Input: dimensioned drawing with shaded views. Units: mm. Origin: part minimum x, y, z. A direction names the side the tool comes from. Give positions to 0.01 mm unless a question says otherwise; leave off trailing zeros. Write each loop counter-clockwise with the first axis right and the second up, starting at its lowest first coordinate (ties: lowest second). Pieces come first, ordered by that corner, then holes.
Q1. Section D-D (x = 37.5). Return the cut outline in (y, z).
Q2. Pin query (flat end, axial travel): pin 1 Ø5 at (y, z) = (12, 67) entering from -X; pin 2 Ø1.5 at (x, y) = (29.5, 11) entering from -Z; pin 3 Ø3 at (x, y) = (45.5, 15.5) entering from +Z; pin 4 Ø10 at (x, y) = (33.5, 15.5) entering from +Z. Return the tip coordinate at first contact, or that it passes through.
Q3. Section A-A (x = 30). Return the cut outline in (y, z), plus the area to 3 significant figures.
Q4. Reachability of the marked faces 1, 2 and 3 from +Z, -Z, +X, -X, +Y, -Y: full face, straight path, thin tool, end or side. Return the list, or none.
Q5. Section C-C (z = 60). Return the cut outline in (x, y).
Q6. Line query: line 1 (Z direction, x = 15, y = 0.35); line 2 (Y direction, x = 49, z = 55); line 3 (Z direction, x = 49, y = 8.5). Output: solid intervals per line, ascending.
Q7. Section B-B (y = 9.25). Return the cut outline in (x, z).
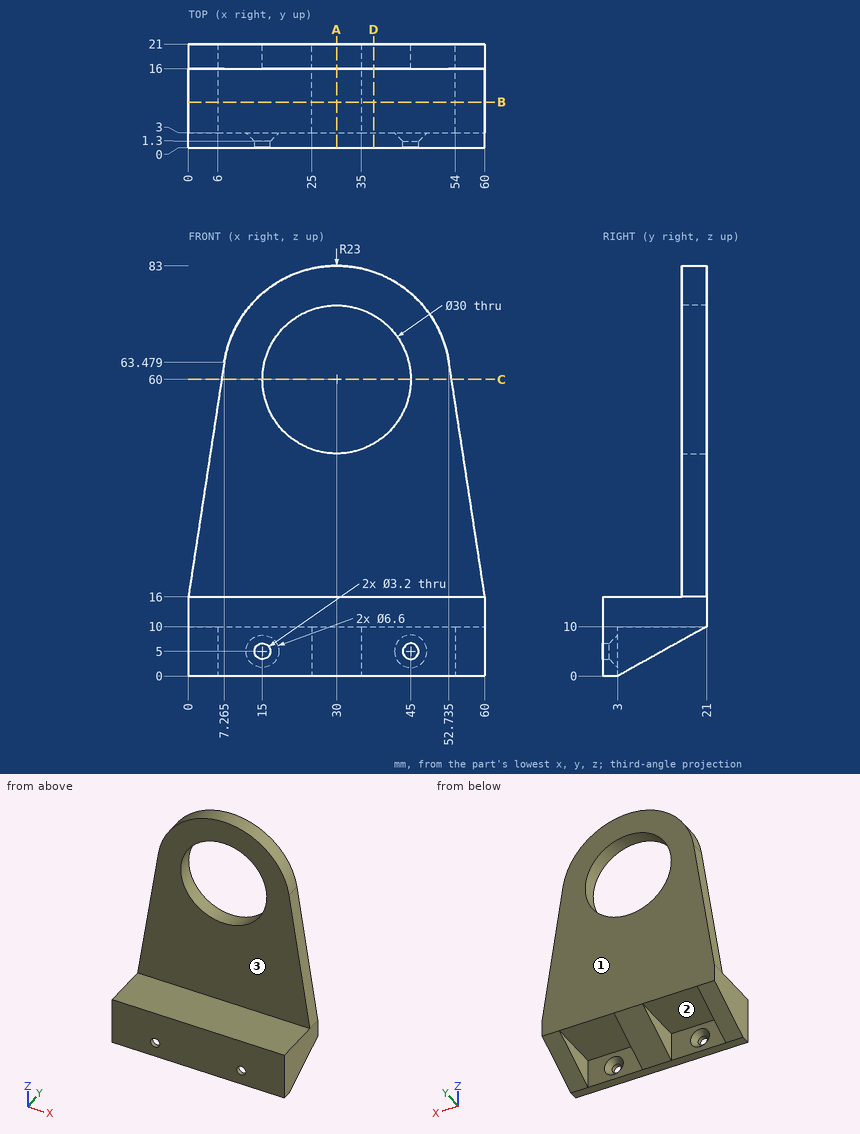
Computed:
1. outline: (0, 0) - (3, 0) - (3, 10) - (21, 10) - (21, 47.01) - (16, 47.01) - (16, 16) - (0, 16) - close; (16, 72.99) - (21, 72.99) - (21, 81.74) - (16, 81.74) - close
2. pin 1: passes through
2. pin 2: stops at z = 4.03
2. pin 3: stops at z = 78.18
2. pin 4: stops at z = 83
3. outline: (0, 0) - (3, 0) - (21, 10) - (21, 45) - (16, 45) - (16, 16) - (0, 16) - close; (16, 75) - (21, 75) - (21, 83) - (16, 83) - close
3. area: 431 mm2
4. face 1: +Z, -Z, +X, -X, +Y
4. face 2: -Z, +Y
4. face 3: +Z, +X, -X, -Y
5. outline: (6.73, 16) - (15, 16) - (15, 21) - (6.73, 21) - close; (45, 16) - (53.27, 16) - (53.27, 21) - (45, 21) - close
6. line 1: z = 0 to 3.4, 6.6 to 16
6. line 2: y = 16 to 21
6. line 3: z = 10 to 16
7. outline: (0, 3.47) - (6, 3.47) - (6, 10) - (25, 10) - (25, 3.47) - (35, 3.47) - (35, 10) - (54, 10) - (54, 3.47) - (60, 3.47) - (60, 16) - (0, 16) - close
